```python
from build123d import *

# Parameters (mm, degrees)
SALIENTE_EXTRUIR1_DEPTH = 9
CROQUIS2_R              = 2
CORTAR_EXTRUIR1_DEPTH   = 10


with BuildPart() as part:
    # Croquis1 → Saliente-Extruir1 (new, symmetric)
    with BuildSketch(Plane.XY):
        with BuildLine():
            Line((-32, 0), (-33, 0))
            ThreePointArc((-33, 0), (0, -33), (33, 0))
            Line((33, 0), (32, 0))
            ThreePointArc((32, 0), (0, -32), (-32, 0))
        make_face()
    extrude(amount=SALIENTE_EXTRUIR1_DEPTH, both=True)

    # Croquis2 → Cortar-Extruir1 (cut)
    with BuildSketch(Plane.XZ.offset(33)):
        with Locations(Location((0, 0, 0), (0, 0, 270))):
            Circle(CROQUIS2_R)
    extrude(amount=-CORTAR_EXTRUIR1_DEPTH, mode=Mode.SUBTRACT)


solid = part.part
```
Part model, mm, in its own coordinate system. Round coordinates to 2 decimals unless told otherwise and drop trailing zeros. Loops run counter-clockwise (first coordinate to the right, second up) from the corner with the lowest first, then second, coordinate; pieces in that order, holes last. Notation, with made-up numbers: (25, -15) -> (38, -15) arc R15 cw to (38, 11) -> close; hole circle Ø6 at (-16.5, 51.25). An arc over 180 degrees is marked (long way). Use a Markdown table: item, result.
1) Cut at D-D, the plane x = -7. List the corners of the cut face in (y, z), and give its area (3 significant figures).
The answers:
| item | result |
|---|---|
| outline | (-32.25, -9) -> (-31.22, -9) -> (-31.22, 9) -> (-32.25, 9) -> close |
| area | 18.4 mm2 |
2) Cut at C-C, the plane z = -4.5. List the corners of the cut face in (x, y), and give its area (3 significant figures).
The answers:
| item | result |
|---|---|
| outline | (-33, 0) arc R33 ccw to (33, 0) -> (32, 0) arc R32 cw to (-32, 0) -> close |
| area | 102 mm2 |
3) Cut at B-B, the plane y = -6. List the corners of the cut face in (x, z), and give its area (3 significant figures).
The answers:
| item | result |
|---|---|
| outline | (-32.45, -9) -> (-31.43, -9) -> (-31.43, 9) -> (-32.45, 9) -> close; (31.43, -9) -> (32.45, -9) -> (32.45, 9) -> (31.43, 9) -> close |
| area | 36.6 mm2 |
4) Pull direction X, two halves, no side cores. Call faces 1 (the cylindrical face through (-0.73, -32.99, 2.13)), 2 (the cylindrical face through (0.704, -31.992, 2.126)), 3 (the cylindrical face through (-0.766, -32.476, -1.847)), 4 (the flat face through (-0.2, -32.3, 9)): pulls with the +X half, pulls with the -X half, needs draft (parallel to the pull), parting line crosses it, or undercut.
The answers:
| item | result |
|---|---|
| face 1 | parting line crosses it |
| face 2 | undercut |
| face 3 | undercut |
| face 4 | needs draft |
5) Probe line 1 (Z direction, x = 0, y = -32.4); line 2 (X direction, y = -23.5, z = -2.5); line 3 (X direction, y = -4, z = 6.25). List the from-to ranges inside material, lowest first. Write a range as [from, to].
The answers:
| item | result |
|---|---|
| line 1 | z = [-9, -2], [2, 9] |
| line 2 | x = [-23.17, -21.72], [21.72, 23.17] |
| line 3 | x = [-32.76, -31.75], [31.75, 32.76] |
6) Cut at A-A, the plane x = 0. List the corners of the cut face in (y, z).
The answers:
| item | result |
|---|---|
| outline | (-33, -9) -> (-32, -9) -> (-32, -2) -> (-33, -2) -> close; (-33, 2) -> (-32, 2) -> (-32, 9) -> (-33, 9) -> close |
7) Drop flat-ended pins along their axis: pin 1 Ø2 at (y, z) = (-6.5, -6) entering from +X; pin 2 Ø8 at (y, z) = (-26.5, 2) entering from -X; pin 3 Ø4 at (y, z) = (-6.5, 1.5) entering from +X; pin 4 Ø12 at (x, y) = (-7.5, -22) entering from -Z. Give the stop position or say it passes through.
The answers:
| item | result |
|---|---|
| pin 1 | stops at x = 32.54 |
| pin 2 | stops at x = -24.14 |
| pin 3 | stops at x = 32.69 |
| pin 4 | passes through |
